Input: part model. Units: mm. Frame: model coordinates. A direction names the side the tool comes from. Coordinates: 2 decimals unless noted, no trailing zeros. Loops run counter-clockwise (first coordinate to the right, second up) from the corner with the lowest first, then second, coordinate; pieces in that order, holes last. Notation, with made-up numbers: M -3,34.5 L 39,34.5 A15 ccw 39,50.5 Z; hole C -32,12 d1. An arc over 180 degrees is marked long. Use a Markdown table: item, result. Add a question column.
1. Pin query (flat end, axial travel): pin 1 (22 mm diameter, centred on x = 7059, z = -10, fed in from +Y); pin 2 (8 mm diameter, centred on y = -1270, z = -12.5, fed in from -X); pin 3 (3 mm diameter, centred on x = 6988, z = -0.5, fed in from -Y). Return the tip coordinate at first contact, or that it passes through.
2. Section D-D on x = 6961.5. Output: boundary loops of the cut face in (y, z).
3. Set-up query: faces 4 (the flat face through (7063, -1280.655, 5)), 5 (the flat face through (7032, -1288.655, 0)), 6 (the flat face through (6997.507, -1273.047, 0.28)). Return all of +Z, -Z, +X, -X, +Y, -Y with unobstructed straight access to the full face (end or side cutting, diameter ignored); none if empty.
4. Section B-B on z = 16. Output: boundary loops of the cut face in (x, y), then the cut area to 3 significant figures.
5. Section A-A on z = -1.5. Output: boundary loops of the cut face in (x, y), then the cut area to 3 significant figures.
6. Line query: L1, parallel to Y at x = 7039, z = 15; L2, parallel to Y at x = 6957.5, z = -6.5; L3, parallel to X at y = -1265, z = -17. Output: solid intervals per line, ascending. Write a range as [from, to].
7. Draft query along X for faces 1 (the cylindrical face through (6997.124, -1278.139, 0.28)), 2 (the flat face through (7004, -1262, -20)), 3 (the flat face through (7072.688, -1285, 0)). Return one class per face: +X half, -X half, draft (parallel to the pull), parting line (faces both ways), or undercut.
8. Section C-C on y = -1247. Output: boundary loops of the cut face in (x, z).
```python
from build123d import *

# Parameters (mm, degrees)
EXTRUDE_1_DEPTH         = 20
HOLE_WIZARD_8_5_8_5_1_D = 8.5
HOLE_WIZARD_8_5_8_5_2_D = 8.5


with BuildPart() as part:
    # 草图1 → 凸台-拉伸1 (new, symmetric)
    with BuildSketch(Plane.XY):
        Polygon((6936.119122288, -1232.086390659), (6992.687664783, -1288.654933154), (7072.687664783, -1288.654933154), (7072.687664783, -1280.654933154), (7052.687664783, -1280.654933154), (6955.918112162, -1240.571672033), (6941.775976538, -1226.429536409), align=None)
        with BuildLine():
            Line((7009.090927681, -1283.654933154), (7003.090927681, -1283.654933154))
            Line((7003.090927681, -1283.654933154), (6999.760549745, -1280.324555218))
            ThreePointArc((6999.760549745, -1280.324555218), (7002.213755914, -1277.239517812), (7001.296666197, -1273.406161221))
            Line((7001.296666197, -1273.406161221), (6999.365595427, -1274.993916141))
            ThreePointArc((6999.365595427, -1274.993916141), (6997.055371947, -1278.111879141), (6997.626530039, -1274.273571671))
            Line((6997.626530039, -1274.273571671), (6997.383769074, -1271.785386165))
            ThreePointArc((6997.383769074, -1271.785386165), (6994.101203016, -1273.731324494), (6993.49338103, -1277.49861375))
            Line((6993.49338103, -1277.49861375), (6988.602413191, -1277.49861375))
            Line((6988.602413191, -1277.49861375), (6954.21874867, -1243.114949228))
            Line((6954.21874867, -1243.114949228), (7052.090927681, -1283.654933154))
            Line((7052.090927681, -1283.654933154), (7029.403393536, -1283.654933154))
            Line((7029.403393536, -1283.654933154), (7009.090927681, -1283.654933154))
        make_face(mode=Mode.SUBTRACT)
    extrude(amount=EXTRUDE_1_DEPTH, both=True)

    # Ø8.5 (8.5) 直径孔1 (through all)
    with Locations(Plane(origin=(2852.016365815, 2852.016365815, 0), x_dir=(0.7071067811865628, -0.7071067811865324, 0), z_dir=(-0.7071067811865324, -0.7071067811865628, 0))):
        with Locations((5785.79350833, 0)):
            Hole(HOLE_WIZARD_8_5_8_5_1_D / 2)

    # Ø8.5 (8.5) 直径孔2 (through all)
    with Locations(Plane.XZ.offset(1288.654933154)):
        with Locations((7062.687664783, 0)):
            Hole(HOLE_WIZARD_8_5_8_5_2_D / 2)


solid = part.part
```
Answers below:
| question | item | result |
|---|---|---|
| 1 | pin 1 | stops at y = -1278.71 |
| 1 | pin 2 | stops at x = 6970.03 |
| 1 | pin 3 | stops at y = -1285.47 |
| 2 | outline | M -1257.47,-20 L -1250.4,-20 L -1250.4,20 L -1257.47,20 Z; M -1246.13,-20 L -1242.88,-20 L -1242.88,20 L -1246.13,20 Z |
| 3 | face 4 | +Z, -Z, +X, +Y |
| 3 | face 5 | +Z, -Z, +X, -X, -Y |
| 3 | face 6 | +Z, -Z |
| 4 | outline | M 6936.12,-1232.09 L 6992.69,-1288.65 L 7072.69,-1288.65 L 7072.69,-1280.65 L 7052.69,-1280.65 L 6955.92,-1240.57 L 6941.78,-1226.43 Z; hole M 6954.22,-1243.11 L 6988.6,-1277.5 L 6993.49,-1277.5 A4.5 cw 6997.38,-1271.79 L 6997.63,-1274.27 A2 ccw long 6999.37,-1274.99 L 7001.3,-1273.41 A4.5 cw 6999.76,-1280.32 L 7003.09,-1283.65 L 7052.09,-1283.65 Z |
| 4 | area | 1,310 mm² |
| 5 | outline | M 6936.12,-1232.09 L 6940.38,-1236.35 L 6946.04,-1230.69 L 6941.78,-1226.43 Z; M 6946,-1241.97 L 6992.69,-1288.65 L 7058.71,-1288.65 L 7058.71,-1280.65 L 7052.69,-1280.65 L 6955.92,-1240.57 L 6951.66,-1236.31 Z; M 7066.66,-1288.65 L 7072.69,-1288.65 L 7072.69,-1280.65 L 7066.66,-1280.65 Z; hole M 6954.22,-1243.11 L 6988.6,-1277.5 L 6993.49,-1277.5 A4.5 cw 6997.38,-1271.79 L 6997.63,-1274.27 A2 ccw long 6999.37,-1274.99 L 7001.3,-1273.41 A4.5 cw 6999.76,-1280.32 L 7003.09,-1283.65 L 7052.09,-1283.65 Z |
| 5 | area | 1,180 mm² |
| 6 | L1 | y = [-1288.65, -1283.65], [-1278.23, -1274.99] |
| 6 | L2 | y = [-1253.47, -1246.4], [-1244.47, -1241.23] |
| 6 | L3 | x = [6969.03, 6976.1], [7007.05, 7014.89] |
| 7 | face 1 | undercut |
| 7 | face 2 | draft |
| 7 | face 3 | +X half |
| 8 | outline | M 6951.03,-20 L 6958.1,-20 L 6958.1,20 L 6951.03,20 Z; M 6963.6,-20 L 6971.44,-20 L 6971.44,20 L 6963.6,20 Z |
